Here's how the part is built. I have some questions about the finished solid (model axes, mm). Face numbers are marked on the shaded views. A direction names the side the tool comes from. Coordinates: 2 decimals unless noted, no trailing zeros. Write each loop counter-clockwise with the first axis right and the second up, starting at its lowest first coordinate (ties: lowest second). Pieces come first, ordered by that corner, then holes.
```python
from build123d import *

# Parameters (mm, degrees)
SKETCH1_W                               = 131
SKETCH1_H                               = 53.5
EXTRUDE1_DEPTH                          = 14
CUT_SWEEP1_START                        = -14
CUT_SWEEP1_OUTLINE_W                    = 105
CUT_SWEEP1_OUTLINE_H                    = 1
CUT_SWEEP1_DEPTH                        = 28
CUT_SWEEP1_2_OUTLINE_W                  = 105
CUT_SWEEP1_2_OUTLINE_H                  = 51.5
CUT_SWEEP1_2_DEPTH                      = 1
CUT_SWEEP1_START_2                      = 13
CUT_SWEEP1_3_OUTLINE_W                  = 105
CUT_SWEEP1_3_OUTLINE_H                  = 51.5
CUT_SWEEP1_3_DEPTH                      = 1
SKETCH3_R                               = 7.6
CUT_EXTRUDE1_DEPTH                      = 135.434231132
CBORE_FOR_M5_HEX_HEAD_BOLT1_D           = 5.5
CBORE_FOR_M5_HEX_HEAD_BOLT1_CBORE_D     = 9
CBORE_FOR_M5_HEX_HEAD_BOLT1_CBORE_DEPTH = 6
CHAMFER1_SIZE                           = 1
M5X0_8_TAPPED_HOLE1_D                   = 4.2
M5X0_8_TAPPED_HOLE1_DEPTH               = 12.4
M5X0_8_TAPPED_HOLE1_TIP                 = 1.2618073


# Read off the part's stored shape, not the designer's step: Cut-Sweep1
with BuildPart() as part:
    # Sketch1 → Extrude1 (new, symmetric)
    with BuildSketch(Plane.XY):
        Rectangle(SKETCH1_W, SKETCH1_H)
    extrude(amount=EXTRUDE1_DEPTH, both=True)

    # Cut-Sweep1 outline → Cut-Sweep1 (cut)
    with BuildSketch(Plane.XY.offset(CUT_SWEEP1_START)):
        with Locations((0, -26.25)):
            Rectangle(CUT_SWEEP1_OUTLINE_W, CUT_SWEEP1_OUTLINE_H)
        with Locations((0, 26.25)):
            Rectangle(CUT_SWEEP1_OUTLINE_W, CUT_SWEEP1_OUTLINE_H)
    extrude(amount=CUT_SWEEP1_DEPTH, mode=Mode.SUBTRACT)

    # Cut-Sweep1 2 outline → Cut-Sweep1 2 (cut)
    with BuildSketch(Plane.XY.offset(CUT_SWEEP1_START)):
        Rectangle(CUT_SWEEP1_2_OUTLINE_W, CUT_SWEEP1_2_OUTLINE_H)
    extrude(amount=CUT_SWEEP1_2_DEPTH, mode=Mode.SUBTRACT)

    # Cut-Sweep1 3 outline → Cut-Sweep1 3 (cut)
    with BuildSketch(Plane.XY.offset(CUT_SWEEP1_START_2)):
        Rectangle(CUT_SWEEP1_3_OUTLINE_W, CUT_SWEEP1_3_OUTLINE_H)
    extrude(amount=CUT_SWEEP1_3_DEPTH, mode=Mode.SUBTRACT)

    # Sketch3 → Cut-Extrude1 (cut, through all)
    with BuildSketch(Plane.ZY.offset(65.5)):
        with Locations(Location((0, 12, 0), (0, 0, 270))):
            Circle(SKETCH3_R)
    extrude(amount=-CUT_EXTRUDE1_DEPTH, mode=Mode.SUBTRACT)

    # CBORE for M5 Hex Head Bolt1 (through all)
    with Locations(Plane(origin=(-59, -6.75, 14), x_dir=(1, 0, 0), z_dir=(0, 0, 1))):
        with Locations((0, 0), (118, 0)):
            CounterBoreHole(CBORE_FOR_M5_HEX_HEAD_BOLT1_D / 2, CBORE_FOR_M5_HEX_HEAD_BOLT1_CBORE_D / 2, CBORE_FOR_M5_HEX_HEAD_BOLT1_CBORE_DEPTH)

    # Chamfer1
    chamfer1_edges = [part.edges().sort_by_distance(p)[0] for p in [
        (65.5, 19.6, 0),
        (-65.5, 19.6, 0),
    ]]
    chamfer(chamfer1_edges, length=CHAMFER1_SIZE)

    # M5x0.8 Tapped Hole1
    with Locations(Plane(origin=(-59, -26.75, -3), x_dir=(0, 0, -1), z_dir=(0, -1, 0))):
        with Locations((0, 0), (0, 118.655251347)):
            Hole(M5X0_8_TAPPED_HOLE1_D / 2, depth=M5X0_8_TAPPED_HOLE1_DEPTH)
            with Locations((0, 0, -(M5X0_8_TAPPED_HOLE1_DEPTH + M5X0_8_TAPPED_HOLE1_TIP / 2))):  # 118° drill point
                Cone(0, M5X0_8_TAPPED_HOLE1_D / 2, M5X0_8_TAPPED_HOLE1_TIP, mode=Mode.SUBTRACT)


solid = part.part
```
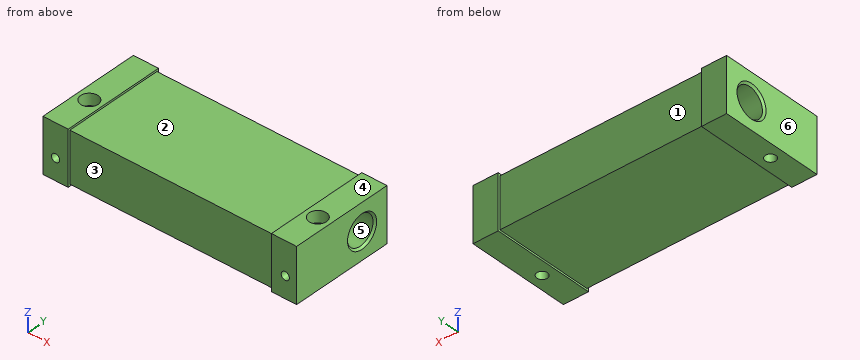
1) On a 3-axis mill with a long thin cutter (end or side, diameter ignored), from which of +Z, -Z, +X, -X, +Y, -Y can I reach the whole of each face in a straight line? I mean the marked faces 1, 2 and 3. Say none if no direction works.
Values follow:
face 1: +Z, -Z, +Y
face 2: +Z, +Y, -Y
face 3: +Z, -Z, -Y
2) Imagine slicing it at D-D on x = 1.5. Please give me the cut outline in (y, z).
Values follow:
outline: (-25.75, -13) - (25.75, -13) - (25.75, 13) - (-25.75, 13) - close; hole circle Ø15.2 at (12, 0)
3) Will these pins go through, and if not, where does the flat tip stop? pin 1 (3 mm diameter, centred on x = -1.5, z = -4.5, fed in from -Y); pin 2 (6.5 mm diameter, centred on x = 59, y = -6.75, fed in from +Z); pin 3 (8 mm diameter, centred on x = 42, y = 21.5, fed in from +Z); pin 4 (3.5 mm diameter, centred on x = -59, y = -6.75, fed in from -Z).
Values follow:
pin 1: stops at y = -25.75
pin 2: stops at z = 8
pin 3: stops at z = 13
pin 4: passes through
4) I need wall thicknesses on probe 1 along Y at (x, z) = (59, 9.4); probe 2 along Y at (x, z) = (59, 3.5); probe 3 along Z at (x, y) = (-13, 12). Which ranges of each line are inside material? Lowest first, please.
Values follow:
probe 1: y = -26.75 to -11.25, -2.25 to 26.75
probe 2: y = -26.75 to -9.5, -4 to 5.25, 18.75 to 26.75
probe 3: z = -13 to -7.6, 7.6 to 13
5) Imagine slicing it at A-A on y = 12. Please give me the cut outline in (x, z).
Values follow:
outline: (-65.5, -14) - (-52.5, -14) - (-52.5, -13) - (52.5, -13) - (52.5, -14) - (65.5, -14) - (65.5, -8.6) - (64.5, -7.6) - (-64.5, -7.6) - (-65.5, -8.6) - close; (-65.5, 8.6) - (-64.5, 7.6) - (64.5, 7.6) - (65.5, 8.6) - (65.5, 14) - (52.5, 14) - (52.5, 13) - (-52.5, 13) - (-52.5, 14) - (-65.5, 14) - close
6) Imagine slicing it at B-B on y = -6.75. Please give me the cut outline in (x, z).
Values follow:
outline: (-65.5, -14) - (-61.75, -14) - (-61.75, 8) - (-63.5, 8) - (-63.5, 14) - (-65.5, 14) - close; (-56.25, -14) - (-52.5, -14) - (-52.5, -13) - (52.5, -13) - (52.5, -14) - (56.25, -14) - (56.25, 8) - (54.5, 8) - (54.5, 14) - (52.5, 14) - (52.5, 13) - (-52.5, 13) - (-52.5, 14) - (-54.5, 14) - (-54.5, 8) - (-56.25, 8) - close; (61.75, -14) - (65.5, -14) - (65.5, 14) - (63.5, 14) - (63.5, 8) - (61.75, 8) - close
7) We'd pull the mould along Z, two halves only. Please class the marked faces 4, 5 and 6: pulls with the +Z half, pulls with the -Z half, needs draft (parallel to the pull), parting line crosses it, or undercut.
Values follow:
face 4: pulls with the +Z half
face 5: undercut
face 6: needs draft
8) Imagine slicing it at C-C on z = -11.25. Please give me the cut outline in (x, y), then the cut area to 3 significant figures.
Values follow:
outline: (-65.5, -26.75) - (-52.5, -26.75) - (-52.5, -25.75) - (52.5, -25.75) - (52.5, -26.75) - (65.5, -26.75) - (65.5, 26.75) - (52.5, 26.75) - (52.5, 25.75) - (-52.5, 25.75) - (-52.5, 26.75) - (-65.5, 26.75) - close; hole circle Ø5.5 at (-59, -6.75); hole circle Ø5.5 at (59, -6.75)
area: 6,750 mm2
